Model file for the job. Use its own axes, mm. Round coordinates to 2 decimals unless told otherwise and drop trailing zeros. Order: outer loops, then holes, each group sorted by start corner. A loop starts at its lowest first (then second) coordinate and runs counter-clockwise, first axis right, second up. Notation, with made-up numbers: (-22, -32) - (-9, -32) arc R15 cw to (-9, -28) - close; hole circle Ø3 at (57, 41). An arc over 180 degrees is marked (long way). Write item = value, one per line.
```python
from build123d import *

# Parameters (mm, degrees)
BOSS_EXTRUDE1_DEPTH       = 6.35
SKETCH4_W                 = 88.9
SKETCH4_H                 = 3.175
CUT_EXTRUDE1_DEPTH        = 378.010361263
CUT_EXTRUDE2_DEPTH        = 378.010361263
CUT_EXTRUDE5_DEPTH        = 378.010361263
CUT_EXTRUDE6_DEPTH        = 378.010361263
SKETCH12_W                = 22.86
SKETCH12_H                = 3.175
SKETCH12_W_2              = 3.175
CUT_EXTRUDE8_DEPTH        = 378.010361263
NYLON_BOLT_CUT_REACH      = 379.01
SKETCH13_R                = 6.35
SKETCH14_R                = 19.05
CUT_EXTRUDE9_DEPTH        = 378.010361263
SKETCH15_R                = 6.35
STATIC_PAYLOAD_BOLT_DEPTH = 378.010361263
CUT_EXTRUDE10_DEPTH       = 378.010361263


with BuildPart() as part:
    # Sketch3 → Boss-Extrude1 (new body)
    with BuildSketch(Plane.XY):
        with BuildLine():
            Line((-317.5, 65.991135768), (-279.4, 0))
            Line((-279.4, 0), (279.4, 0))
            Line((279.4, 0), (317.5, 65.991135768))
            Line((317.5, 65.991135768), (238.282425301, 203.2))
            Line((238.282425301, 203.2), (218.930796924, 203.2))
            ThreePointArc((218.930796924, 203.2), (194.958955891, 113.108264062), (110.49, 73.66))
            ThreePointArc((110.49, 73.66), (47.902002926, 93.167184987), (7.48041253, 144.78))
            Line((7.48041253, 144.78), (-7.48041253, 144.78))
            ThreePointArc((-7.48041253, 144.78), (-47.902002926, 93.167184987), (-110.49, 73.66))
            ThreePointArc((-110.49, 73.66), (-194.958955891, 113.108264062), (-218.930796924, 203.2))
            Line((-218.930796924, 203.2), (-238.282425301, 203.2))
            Line((-238.282425301, 203.2), (-317.5, 65.991135768))
        make_face()
    extrude(amount=BOSS_EXTRUDE1_DEPTH)

    # Sketch4 → Cut-Extrude1 (cut, through all)
    with BuildSketch(Plane.XY.offset(6.35)):
        with Locations((-209.55, 1.5875)):
            Rectangle(SKETCH4_W, SKETCH4_H)
        with Locations((-69.85, 1.5875)):
            Rectangle(SKETCH4_W, SKETCH4_H)
        with Locations((69.85, 1.5875)):
            Rectangle(SKETCH4_W, SKETCH4_H)
        with Locations((209.55, 1.5875)):
            Rectangle(SKETCH4_W, SKETCH4_H)
    extrude(amount=-CUT_EXTRUDE1_DEPTH, mode=Mode.SUBTRACT)

    # Sketch5 → Cut-Extrude2 (cut, through all)
    with BuildSketch(Plane.XY.offset(6.35)):
        Polygon((-311.15, 54.99261314), (-309.775184671, 55.78636314), (-284.375184671, 11.792272628), (-285.75, 10.998522628), align=None)
        Polygon((285.75, 10.998522628), (311.15, 54.99261314), (309.775184671, 55.78636314), (284.375184671, 11.792272628), align=None)
    extrude(amount=-CUT_EXTRUDE2_DEPTH, mode=Mode.SUBTRACT)

    # Sketch8 → Cut-Extrude5 (cut, through all)
    with BuildSketch(Plane.XY.offset(6.35)):
        Polygon((-315.363184671, 66.517208484), (-236.449338196, 203.2), (-238.282425301, 203.2), (-316.738, 67.310958484), align=None)
        Polygon((316.738, 67.310958484), (315.363184671, 66.517208484), (236.449338196, 203.2), (238.282425301, 203.2), align=None)
    extrude(amount=-CUT_EXTRUDE5_DEPTH, mode=Mode.SUBTRACT)

    # Sketch9 → Cut-Extrude6 (cut, through all)
    with BuildSketch(Plane.XY.offset(6.35)):
        Polygon((-252.959338196, 174.603841167), (-247.460076882, 171.428841167), (-244.285076882, 176.928102481), (-249.784338196, 180.103102481), align=None)
        Polygon((249.784338196, 180.103102481), (252.959338196, 174.603841167), (247.460076882, 171.428841167), (244.285076882, 176.928102481), align=None)
        Polygon((-303.640923357, 74.120760659), (-300.465923357, 79.620021973), (-305.965184671, 82.795021973), (-309.140184671, 77.295760659), align=None)
        Polygon((305.965184671, 82.795021973), (309.140184671, 77.295760659), (303.640923357, 74.120760659), (300.465923357, 79.620021973), align=None)
    extrude(amount=-CUT_EXTRUDE6_DEPTH, mode=Mode.SUBTRACT)

    # Sketch12 → Cut-Extrude8 (cut, through all)
    with BuildSketch(Plane.XY.offset(6.35)):
        with Locations((-130.048, 4.7625)):
            Rectangle(SKETCH12_W, SKETCH12_H)
        with Locations((130.048, 4.7625)):
            Rectangle(SKETCH12_W, SKETCH12_H)
        with Locations((0, 4.7625)):
            Rectangle(SKETCH12_W_2, SKETCH12_H)
    extrude(amount=-CUT_EXTRUDE8_DEPTH, mode=Mode.SUBTRACT)

    # Sketch13 → nylon bolt cut (cut, up to next)
    with BuildSketch(Plane(origin=(0, 0, 0), x_dir=(-1, 0, 0), z_dir=(0, 0, -1)), mode=Mode.PRIVATE) as nylon_bolt_cut_sk1:
        with Locations((-247.65, 80.01)):
            Circle(SKETCH13_R)
    nylon_bolt_cut_tool1 = extrude(nylon_bolt_cut_sk1.sketch, amount=-NYLON_BOLT_CUT_REACH, mode=Mode.PRIVATE) & part.part
    # Sketch13 → nylon bolt cut (cut, up to next)
    with BuildSketch(Plane(origin=(0, 0, 0), x_dir=(-1, 0, 0), z_dir=(0, 0, -1)), mode=Mode.PRIVATE) as nylon_bolt_cut_sk2:
        with Locations(Location((247.65, 80.01, 0), (0, 0, 180))):
            Circle(SKETCH13_R)
    nylon_bolt_cut_tool2 = extrude(nylon_bolt_cut_sk2.sketch, amount=-NYLON_BOLT_CUT_REACH, mode=Mode.PRIVATE) & part.part
    add(nylon_bolt_cut_tool1.solids().sort_by_distance((247.65, 80.01, 0))[0], mode=Mode.SUBTRACT)
    add(nylon_bolt_cut_tool2.solids().sort_by_distance((-247.65, 80.01, 0))[0], mode=Mode.SUBTRACT)

    # Sketch14 → Cut-Extrude9 (cut, through all)
    with BuildSketch(Plane.XY.offset(6.35)):
        with Locations((-247.65, 118.11)):
            Circle(SKETCH14_R)
        with Locations(Location((247.65, 118.11, 0), (0, 0, 180))):
            Circle(SKETCH14_R)
    extrude(amount=-CUT_EXTRUDE9_DEPTH, mode=Mode.SUBTRACT)

    # Sketch15 → static payload bolt (cut, through all)
    with BuildSketch(Plane.XY.offset(6.35)):
        with Locations((0, 113.03)):
            Circle(SKETCH15_R)
    extrude(amount=-STATIC_PAYLOAD_BOLT_DEPTH, mode=Mode.SUBTRACT)

    # Sketch16 → Cut-Extrude10 (cut, through all)
    with BuildSketch(Plane.XY.offset(6.35)):
        with BuildLine():
            Line((-250.19, 41.275), (-29.21, 41.275))
            ThreePointArc((-29.21, 41.275), (-26.515923164, 40.159076836), (-25.4, 37.465))
            Line((-25.4, 37.465), (-25.4, 32.385))
            ThreePointArc((-25.4, 32.385), (-26.515923164, 29.690923164), (-29.21, 28.575))
            Line((-29.21, 28.575), (-250.19, 28.575))
            ThreePointArc((-250.19, 28.575), (-252.884076836, 29.690923164), (-254, 32.385))
            Line((-254, 32.385), (-254, 37.465))
            ThreePointArc((-254, 37.465), (-252.884076836, 40.159076836), (-250.19, 41.275))
        make_face()
        with BuildLine():
            Line((254, 37.465), (254, 32.385))
            ThreePointArc((254, 32.385), (252.884076836, 29.690923164), (250.19, 28.575))
            Line((250.19, 28.575), (29.21, 28.575))
            ThreePointArc((29.21, 28.575), (26.515923164, 29.690923164), (25.4, 32.385))
            Line((25.4, 32.385), (25.4, 37.465))
            ThreePointArc((25.4, 37.465), (26.515923164, 40.159076836), (29.21, 41.275))
            Line((29.21, 41.275), (250.19, 41.275))
            ThreePointArc((250.19, 41.275), (252.884076836, 40.159076836), (254, 37.465))
        make_face()
    extrude(amount=-CUT_EXTRUDE10_DEPTH, mode=Mode.SUBTRACT)


solid = part.part
```
1) Cut at A-A (x = -43). Write the cut outline in (y, z) (3 decimals).
Conclusion:
outline = (3.175, 0) - (28.575, 0) - (28.575, 6.35) - (3.175, 6.35) - close; (41.275, 0) - (96.755, 0) - (96.755, 6.35) - (41.275, 6.35) - close
2) Cut at C-C (z = 3.25). Give the number of separate pieces and of enclosed holes in the cut face, and give its area (3 significant figures).
Conclusion:
separate_pieces = 1
enclosed_holes = 10
area = 58,200 mm^2
3) Flat gauge pins, fed straight in: pin 1 Ø1 at (y, z) = (4.5, 4) entering from +X; pin 2 Ø3.5 at (x, z) = (-0.5, 2.5) entering from +Y; pin 3 Ø1.6 at (y, z) = (2, 2) entering from +X. Where does each tip first touch, or does it go through?
Conclusion:
pin_1 = 282.29
pin_2 = 144.78
pin_3 = 281.02
4) Cut at B-B (y = 163). Write the cut outline in (x, z).
Conclusion:
outline = (-259.66, 0) - (-218.66, 0) - (-218.66, 6.35) - (-259.66, 6.35) - close; (218.66, 0) - (259.66, 0) - (259.66, 6.35) - (218.66, 6.35) - close
5) Wall check: line 1 along Y through (x, z) = (244, 1.5) (3 decimals); line 2 along X through (y, z) = (133, 0.75); line 3 along X through (y, z) = (154, 1.75). Give the ranges that are in metal, low to high.
Conclusion:
line_1 = 3.175 to 28.575, 41.275 to 74.814, 85.206 to 99.413, 136.807 to 190.122
line_2 = -276.98 to -259.53, -235.77 to -208.23, -12.75 to 12.75, 208.23 to 235.77, 259.53 to 276.98
line_3 = -264.85 to -216.54, 216.54 to 264.85
6) Cut at D-D (x = 273). Write the cut outline in (y, z).
Conclusion:
outline = (0, 0) - (139.89, 0) - (139.89, 6.35) - (0, 6.35) - close
